Part model, mm, in its own coordinate system. Face numbers are marked on the shaded views. A direction names the side the tool comes from. Coordinates: 2 decimals unless noted, no trailing zeros. Write each loop counter-clockwise with the first axis right and the second up, starting at its lowest first coordinate (ties: lowest second). Pieces come first, ordered by that corner, then holes. Notation, with made-up numbers: (20, -37.75) -> (30, -37.75) arc R20 cw to (30, -14.75) -> close; hole circle Ø11 at (-12.5, 32.25). An arc over 180 degrees is marked (long way). Write item = value, one per line. Start each with the question number.
Q1. Band-saw the part on A-A, the plane x = -1.5. List the corners of the cut face in (y, z) (3 decimals).
Q2. Band-saw the part on D-D, the plane x = -0.5. List the corners of the cut face in (y, z) (3 decimals), plus the area to 3 significant figures.
Q3. Band-saw the part on C-C, the plane y = 1.2. List the corners of the cut face in (x, z) (3 decimals).
Q4. Probe line 1 (Y direction, x = 2.5, z = -4.5); line 2 (Y direction, x = -2.75, z = -4.25); line 3 (Z direction, x = 2, y = 0.95) (3 decimals). List the from-to ranges inside material, lowest first.
Q5. Tool access for the marked faces 1, 2, 3, 4 and 5: list every direction of +Z, -Z, +X, -X, +Y, -Y with a clear straight run to the whole face (end or side of a thin tool).
Q6. Pin check, flat tips, straight feed: P1, Ø4, axis at x = 2.5, z = -4.5, coming from the +Y side; P2, Ø0.5, axis at y = 0.5, z = -1, coming from the -X side; P3, Ø1.5, axis at x = -1, z = -6.5, coming from the -Y side. Stop position of each tip, or through.
Q7. Pull direction Y, two halves, no side cores. Call the marked faces 6, 7, 8 and 9: released by +Y, released by -Y, zero draft, split by the parting line, or undercut.
Q8. Band-saw the part on B-B, the plane z = 5.5. List the corners of the cut face in (x, y), plus the area to 4 significant figures.
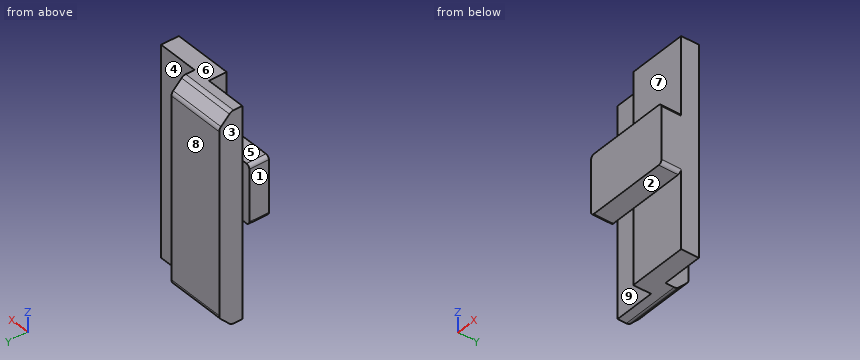
Autodesk Fusion 360 part; units mm, degrees
sketch "Sketch1" plane through (0, 0, 0) normal (0, 1, 0) x (1, 0, 0)
  line L0 (3.68, -2.475) -> (-3.68, -2.475)
  line L1 (-3.68, -2.475) -> (-3.68, 2.475)
  line L2 (-3.68, 2.475) -> (3.68, 2.475)
  line L3 (3.68, 2.475) -> (3.68, -2.475)
  line L4 (3.68, -2.475) -> (-3.68, 2.475) construction
  line L5 (-3.68, -2.475) -> (3.68, 2.475) construction
  dimension "d124" = 7.36
  dimension "d125" = 4.95
extrude "Extrude1" add sketch "Sketch1" along normal blind 1.65 makes body 1
fillet "Fillet1" radius 0.3 4 edges at (-3.68, 0.825, 2.475) (3.68, 0.825, 2.475) (3.68, 0.825, -2.475) (-3.68, 0.825, -2.475) on bodies 1
sketch "Sketch2" plane through (0, 1.65, 0) normal (0, 1, 0) x (-1, 0, 0)
  line L0 (1.32, 8.795) -> (-3.68, 8.795)
  line L1 (-3.68, 8.795) -> (-3.68, -8.795)
  line L2 (-3.68, -8.795) -> (1.32, -8.795)
  line L3 (1.32, -8.795) -> (1.32, 8.795)
  line L4 (-3.68, 2.175) -> (-3.68, -2.175)
  line L5 (0, 0) -> (-3.68, 0) construction
  dimension "d136" = 17.59
  dimension "d137" = 5
extrude "Extrude5" add sketch "Sketch2" along normal blind 1.5 bodies 1
sketch "Sketch6" plane through (0, 3.15, 0) normal (0, 1, 0) x (-1, 0, 0)
  line L0 (-3.68, 8.795) -> (-3.68, -8.795)
  line L1 (-3.68, -8.795) -> (1.32, -8.795)
  line L2 (1.32, -8.795) -> (1.32, 8.795)
  line L3 (1.32, 8.795) -> (-3.68, 8.795)
  line L4 (-0.18, 8.795) -> (4.82, 8.795)
  line L5 (4.82, 8.795) -> (4.82, -8.795)
  line L6 (4.82, -8.795) -> (-0.18, -8.795)
  line L7 (-0.18, -8.795) -> (-0.18, 8.795)
  dimension "d158" = 3.5
extrude "Extrude7" add sketch "Sketch6" along normal blind 1.95 separate body contours L1 L2 L3 L4 L6 L7 | L2 L4 L5 L6 makes body 2
chamfer "Chamfer2" distance 1 angle 45 2 edges at (-2.32, 5.1, 8.795) (-2.32, 5.1, -8.795) on bodies 2
fillet "Fillet3" radius 0.5 4 edges at (-2.32, 5.1, 7.795) (-2.32, 4.1, 8.795) (-2.32, 5.1, -7.795) (-2.32, 4.1, -8.795) on bodies 2
combine "Combine1" operation add target body 2 tool bodies 1
sketch "Sketch7" plane through (0, 0, 0) normal (0, -1, 0) x (1, 0, 0)
  arc A0 (-3.68, -2.175) -> (-3.38, -2.475) centre (-3.38, -2.175) ccw
  line L0 (-3.38, -2.475) -> (3.38, -2.475)
  arc A1 (3.38, -2.475) -> (3.68, -2.175) centre (3.38, -2.175) ccw
  line L1 (3.68, -2.175) -> (3.68, 2.175)
  arc A2 (3.68, 2.175) -> (3.38, 2.475) centre (3.38, 2.175) ccw
  line L2 (3.38, 2.475) -> (-3.38, 2.475)
  arc A3 (-3.38, 2.475) -> (-3.68, 2.175) centre (-3.38, 2.175) ccw
  line L3 (-3.68, 2.175) -> (-3.68, -2.175)
extrude "Extrude8" [suppressed]
equation "d131 = DetentBottomPieceFilletRadius"
equation "d158 = DetentShiftDistance"
equation "DetentBottomPieceFilletRadius = 0.3 mm"
equation "DetentShiftDistance = 3.5 mm"
Ans:
q1.outline = (0, -2.475) -> (1.65, -2.475) -> (1.65, 2.475) -> (0, 2.475) -> close; (3.15, -8.795) -> (3.893, -8.795) arc R0.5 ccw to (4.246, -8.649) -> (4.954, -7.941) arc R0.5 ccw to (5.1, -7.588) -> (5.1, 7.588) arc R0.5 ccw to (4.954, 7.941) -> (4.246, 8.649) arc R0.5 ccw to (3.893, 8.795) -> (3.15, 8.795) -> close
q2.outline = (0, -2.475) -> (1.65, -2.475) -> (1.65, -8.795) -> (3.893, -8.795) arc R0.5 ccw to (4.246, -8.649) -> (4.954, -7.941) arc R0.5 ccw to (5.1, -7.588) -> (5.1, 7.588) arc R0.5 ccw to (4.954, 7.941) -> (4.246, 8.649) arc R0.5 ccw to (3.893, 8.795) -> (1.65, 8.795) -> (1.65, 2.475) -> (0, 2.475) -> close
q2.area = 67.8 mm2
q3.outline = (-3.68, -2.175) arc R0.3 ccw to (-3.38, -2.475) -> (3.38, -2.475) arc R0.3 ccw to (3.68, -2.175) -> (3.68, 2.175) arc R0.3 ccw to (3.38, 2.475) -> (-3.38, 2.475) arc R0.3 ccw to (-3.68, 2.175) -> close
q4.line_1 = 1.65 to 3.15
q4.line_2 = 3.15 to 5.1
q4.line_3 = -2.475 to 2.475
q5.face_1 = +Z, -Z, -X, -Y
q5.face_2 = -Z, +X, -X, -Y
q5.face_3 = +Z, -Z, -X, +Y, -Y
q5.face_4 = +Z, -Z, +X, +Y
q5.face_5 = +Z, +X, -X, -Y
q6.P1 = 3.15
q6.P2 = -3.68
q6.P3 = 1.65
q7.face_6 = zero draft
q7.face_7 = released by -Y
q7.face_8 = released by +Y
q7.face_9 = undercut
q8.outline = (-4.82, 3.15) -> (-1.32, 3.15) -> (-1.32, 1.65) -> (3.68, 1.65) -> (3.68, 3.15) -> (0.18, 3.15) -> (0.18, 5.1) -> (-4.82, 5.1) -> close
q8.area = 17.25 mm2
